Input: part model. Units: mm. Frame: model coordinates. A direction names the side the tool comes from. Coordinates: 2 decimals unless noted, no trailing zeros. Order: outer loops, then holes, each group sorted by start corner. A loop starts at its lowest first (then second) coordinate and runs counter-clockwise, first axis right, second up.
from build123d import *

# Parameters (mm, degrees)
SKETCH1_R           = 8.5
BASE_DEPTH          = 18
BACK_CUT_DEPTH      = 15
BOSS_EXTRUDE2_DEPTH = 45
SKETCH5_R           = 8.5
BOSS_EXTRUDE4_DEPTH = 12
FILLET1_R           = 15
CUT_EXTRUDE2_START  = -24
CUT_EXTRUDE2_DEPTH  = 24


# Read off the part's stored shape, not the designer's step: Boss-Extrude2
with BuildPart() as part:
    # Sketch1 → base (new body)
    with BuildSketch(Plane.XY):
        with BuildLine():
            Line((-95, -35), (0, -35))
            ThreePointArc((0, -35), (31.658229663, -14.925029132), (27, 22.271057451))
            Line((27, 22.271057451), (27, 74))
            ThreePointArc((27, 74), (12.653359163, 97.8514675), (-15.140185324, 96.355643322))
            Line((-15.140185324, 96.355643322), (-114.626166161, 28.97953764))
            ThreePointArc((-114.626166161, 28.97953764), (-128.461050621, -10.26440896), (-95, -35))
        make_face()
        with Locations((0, 74)):
            Circle(SKETCH1_R, mode=Mode.SUBTRACT)
    extrude(amount=BASE_DEPTH)

    # Sketch3 → back cut (cut)
    with BuildSketch(Plane(origin=(0, 0, 0), x_dir=(-1, 0, 0), z_dir=(0, 0, -1))):
        with BuildLine():
            Line((0.568421053, 17.991022692), (95.473684211, 14.99251891))
            ThreePointArc((95.473684211, 14.99251891), (110, 0), (95.473684211, -14.99251891))
            Line((95.473684211, -14.99251891), (0.568421053, -17.991022692))
            ThreePointArc((0.568421053, -17.991022692), (-18, 0), (0.568421053, 17.991022692))
        make_face()
    extrude(amount=-BACK_CUT_DEPTH, mode=Mode.SUBTRACT)

    # Boss-Extrude2 outline → Boss-Extrude2 (add)
    with BuildSketch(Plane.XY.offset(18)):
        with BuildLine():
            Line((-94.999999851, -34.999927116), (0, -35))
            ThreePointArc((0, -35), (35, 0), (0, 35))
            Line((0, 35), (-94.928572613, 35))
            ThreePointArc((-94.928572613, 35), (-129.928554392, 0.035713638), (-94.999999851, -34.999927116))
        make_face()
    extrude(amount=BOSS_EXTRUDE2_DEPTH)

    # Sketch5 → Boss-Extrude4 (add)
    with BuildSketch(Plane.XY.offset(18)):
        with BuildLine():
            Line((-27, 74), (-27, 35))
            Line((-27, 35), (0, 35))
            ThreePointArc((0, 35), (14.925029132, 31.658229663), (27, 22.271057451))
            Line((27, 22.271057451), (27, 74))
            ThreePointArc((27, 74), (0, 101), (-27, 74))
        make_face()
        with Locations((0, 74)):
            Circle(SKETCH5_R, mode=Mode.SUBTRACT)
    extrude(amount=BOSS_EXTRUDE4_DEPTH)

    # Fillet1
    fillet1_edges = [part.edges().sort_by_distance(p)[0] for p in [
        (-27, 35, 24),
    ]]
    fillet(fillet1_edges, radius=FILLET1_R)

    # Sketch6 → Cut-Extrude2 (cut)
    with BuildSketch(Plane.XY.offset(63).offset(CUT_EXTRUDE2_START)):
        with BuildLine():
            Line((-95.473684211, 14.99251891), (-0.568421053, 17.991022692))
            ThreePointArc((-0.568421053, 17.991022692), (18, 0), (-0.568421053, -17.991022692))
            Line((-0.568421053, -17.991022692), (-95.473684211, -14.99251891))
            ThreePointArc((-95.473684211, -14.99251891), (-110, 0), (-95.473684211, 14.99251891))
        make_face()
    extrude(amount=CUT_EXTRUDE2_DEPTH, mode=Mode.SUBTRACT)


solid = part.part
Item 1: Access query for faces 1 (the face through (-129.92, 0.8, 40.18)), 2 (the face through (-47, 35, 40)), 3 (the face through (27, 48, 15)), 4 (the face through (18, 0, 51)), 5 (the face through (-110, 0, 7)). Directions: +Z, -Z, +X, -X, +Y, -Y. A direction counts if a zero-diameter tool reaches every point of the face in a straight line with its end or side. Return the directions, or none.
Response values:
face 1: +Z, -X
face 2: +Z, -X, +Y
face 3: +Z, -Z, +X, +Y
face 4: +Z
face 5: -Z
Item 2: Pin query (flat end, axial travel): pin 1 Ø9 at (y, z) = (36.5, 19.5) entering from +X; pin 2 Ø11 at (x, y) = (-50, 1) entering from -Z; pin 3 Ø13.5 at (x, y) = (0, 74) entering from +Z; pin 4 Ø4 at (x, z) = (-59, 25.5) entering from +Y. Return the tip coordinate at first contact, or that it passes through.
Response values:
pin 1: stops at x = 27
pin 2: stops at z = 15
pin 3: passes through
pin 4: stops at y = 35
Item 3: Cut plane C-C on y = 0. Return loops of the section in (x, z).
Response values:
outline: (-130, 0) - (-110, 0) - (-110, 15) - (18, 15) - (18, 0) - (35, 0) - (35, 63) - (18, 63) - (18, 39) - (-110, 39) - (-110, 63) - (-129.93, 63) - (-129.93, 18) - (-130, 18) - close
Item 4: Cut plane A-A on z = 44. Return loops of the section in (x, y), then the cut area to 3 significant figures.
Response values:
outline: (-95, -35) - (0, -35) arc R35 ccw to (0, 35) - (-94.93, 35) arc R35 ccw to start; hole (-95.47, -14.99) - (-0.57, -17.99) arc R18 ccw (long way) to (-0.57, 17.99) - (-95.47, 14.99) arc R15 ccw to start
area: 6,490 mm2
Item 5: Ray query, probe 1 along Y at (x, z) = (0, 23); probe 2 along X at (y, z) = (1, 6.5); probe 3 along X at (y, z) = (0, 56.5). Return the intervals inside material, ascending.
Response values:
probe 1: y = -35 to 65.5, 82.5 to 101
probe 2: x = -129.99 to -109.97, 17.97 to 34.99
probe 3: x = -129.93 to -110, 18 to 35
Item 6: Draft query along Y for faces 6 (the face through (-64.187, 63.139, 8.874)), 7 (the face through (-30, 34, 0)), 8 (the face through (-1.107, 82.428, 14.79)), 9 (the face through (-48, -35, 9)). Return one class per face: pulls with the +Y half, pulls with the -Y half, needs draft (parallel to the pull), parting line crosses it, or undercut.
Response values:
face 6: pulls with the +Y half
face 7: needs draft
face 8: undercut
face 9: pulls with the -Y half
Item 7: Cut plane B-B on x = 5. Return loops of the section in (y, z).
Response values:
outline: (-34.64, 0) - (-17.29, 0) - (-17.29, 15) - (17.29, 15) - (17.29, 0) - (67.13, 0) - (67.13, 30) - (34.64, 30) - (34.64, 63) - (17.29, 63) - (17.29, 39) - (-17.29, 39) - (-17.29, 63) - (-34.64, 63) - close; (80.87, 0) - (100.53, 0) - (100.53, 30) - (80.87, 30) - close
